from build123d import *

# Parameters (mm, degrees)
F0_W     = 50.8
F0_H     = 38.1
F1_DEPTH = 31.75
F3_DEPTH = 50.801
F4_W     = 25.4
F4_H     = 19.05
F5_DEPTH = 31.751


with BuildPart() as f1:
    # F0 (on Front) → F1 (new body)
    with BuildSketch(Plane.XZ):
        with Locations((-34.38605, 26.091824)):
            Rectangle(F0_W, F0_H)
    extrude(amount=F1_DEPTH)

    # F2 (on face) → F3 (cut, through all)
    with BuildSketch(Plane.YZ.offset(-8.98605)):
        with BuildLine():
            Line((-31.75, 45.141824), (-31.75, 19.741824))
            ThreePointArc((-31.75, 19.741824), (-16.111006, 29.50283), (-6.35, 45.141824))
            Line((-6.35, 45.141824), (-31.75, 45.141824))
        make_face()
    extrude(amount=-F3_DEPTH, mode=Mode.SUBTRACT)

    # F4 (on face) → F5 (cut, through all)
    with BuildSketch(Plane(origin=(0, 0, 0), x_dir=(-1, 0, 0), z_dir=(0, 1, 0))):
        with Locations((34.38605, 35.616824)):
            Rectangle(F4_W, F4_H)
    extrude(amount=-F5_DEPTH, mode=Mode.SUBTRACT)


solid = f1.part
CAD build for the part. Positions are in the model's coordinates, mm. A direction names the side the tool comes from. Coordinates: 2 decimals unless noted, no trailing zeros. Loops run counter-clockwise (first coordinate to the right, second up) from the corner with the lowest first, then second, coordinate; pieces in that order, holes last. Notation, with made-up numbers: (85.25, -10) - (97.25, -10) arc R17 cw to (97.25, -2) - close; hole circle Ø4 at (30.25, 35). An arc over 180 degrees is marked (long way). Write item = value, one per line. Start each with the question number.
Q1. Which spindle directions (+Z, -Z, +X, -X, +Y, -Y) get a long thin tool onto all of the face, cutting with end or side? Do faces 1 (the flat face through (-35, -31.75, 13)), 2 (the flat face through (-47.086, -8, 33)). Say none if no direction does.
Q2. Flat gauge pin, fed straight in: pin 1 Ø12 at (x, y) = (-31.5, -23.5) entering from +Z. Where does the tip first touch, or does it go through?
Q3. Cut at D-D, the plane x = -41. List the corners of the cut face in (y, z), then the cut area to 3 significant figures.
Q4. Cut at A-A, the plane z = 38. List the corners of the cut face in (x, y), then the cut area to 3 significant figures.
Q5. Cut at B-B, the plane y = -3.5. List the corners of the cut face in (x, z), then the cut area to 3 significant figures.
Q6. Pull direction X, two halves, no side cores. Call faces 3 (the flat face through (-21.686, -8, 33)), 4 (the flat face through (-54, -3, 45.142)), 5 (the flat face through (-59.786, -12, 22)), 6 (the flat face through (-34, -10, 26.092)): pulls with the +X half, pulls with the -X half, needs draft (parallel to the pull), parting line crosses it, or undercut.
Q7. Drill centre lines: L1, parallel to X at y = -17, z = 28.5; L2, parallel to Y at x = -29.5, z = 26; L3, parallel to Y at x = -54.5, z = 43.5. Where is each one in solid material? Low to high.
Q8. Cut at C-C, the plane x = -48. List the corners of the cut face in (y, z).
Computed:
q1.face_1 = +Z, -Z, +X, -X, -Y
q1.face_2 = +Z, +Y, -Y
q2.pin_1 = 26.09
q3.outline = (-31.75, 7.04) - (0, 7.04) - (0, 26.09) - (-19.98, 26.09) arc R40.88 cw to (-31.75, 19.74) - close
q3.area = 563 mm²
q4.outline = (-59.79, -9.6) - (-47.09, -9.6) - (-47.09, 0) - (-59.79, 0) - close; (-21.69, -9.6) - (-8.99, -9.6) - (-8.99, 0) - (-21.69, 0) - close
q4.area = 244 mm²
q5.outline = (-59.79, 7.04) - (-8.99, 7.04) - (-8.99, 45.14) - (-21.69, 45.14) - (-21.69, 26.09) - (-47.09, 26.09) - (-47.09, 45.14) - (-59.79, 45.14) - close
q5.area = 1,450 mm²
q6.face_3 = undercut
q6.face_4 = needs draft
q6.face_5 = pulls with the -X half
q6.face_6 = undercut
q7.L1 = -59.79 to -47.09, -21.69 to -8.99
q7.L2 = -20.1 to 0
q7.L3 = -6.95 to 0
q8.outline = (-31.75, 7.04) - (0, 7.04) - (0, 45.14) - (-6.35, 45.14) arc R40.88 cw to (-31.75, 19.74) - close
